Here's how the part is built. I have some questions about the finished solid (model axes, mm). Round coordinates to 2 decimals unless told otherwise and drop trailing zeros. Write each loop counter-clockwise with the first axis right and the second up, starting at its lowest first coordinate (ties: lowest second). Pieces come first, ordered by that corner, then holes. Notation, with made-up numbers: (51.5, 28.5) - (91.5, 28.5) arc R19 ccw to (91.5, 40.5) - close; hole circle Ø6 at (87, 88). An arc over 180 degrees is marked (long way). One line per item, written item: value. Start each with the question number.
Item 1: Imagine slicing it at A-A, the plane x = 0. Please give me the cut outline in (y, z), then the cut area to 3 significant figures.
Item 2: For P1, Ø4, axis at x = -10, z = 3, coming from the -Y side; P2, Ø3, axis at y = -8.5, z = 0, coming from the +X side; P3, Ø2, axis at x = 1, y = -11, coming from the +Z side, each with a flat end and sliding along its axis, tell me the tip position at first contact or that it passes through.
Item 3: Imagine slicing it at C-C, the plane z = -7. Please give me the cut outline in (x, y), then the cut area to 3 significant figures.
Item 4: Thinking about a two-plate mould opening in Y: for faces 1 (the face through (-7.78, 4.05, -10.34)), 2 (the face through (-10.144, -2.253, -11.037)), 3 (the face through (-6, -6, -1.149)), which applies, released by +Y, released by -Y, zero draft, split by the parting line, or undercut?
Item 5: If I drill on line 1 (Z direction, x = 18, y = 13.5); line 2 (X direction, y = 1, z = -15.5); line 3 (Y direction, x = -7, z = -20.5), over which ranges is the centre line in solid material (lowest first)?
Item 6: Imagine slicing it at D-D, the plane z = 9.5. Please give me the cut outline in (x, y).
Autodesk Inventor part; units mm, degrees
ref_plane "YZ Plane" through (0, 0, 0) normal (1, 0, 0) x (0, 1, 0)
ref_plane "XZ Plane" through (0, 0, 0) normal (0, 1, 0) x (-1, 0, 0)
ref_plane "XY Plane" through (0, 0, 0) normal (0, 0, 1) x (1, 0, 0)
sketch "Sketch1" plane through (0, 0, 0) normal (1, 0, 0) x (0, 1, 0)
  line L0 (22, 22.8504) -> (6, 0)
  line L1 (6, 0) -> (13, -26.1244)
  line L2 (13, -26.1244) -> (14.4343, -26.1244)
  line L3 (14.4343, -26.1244) -> (7.7423, -1.1493)
  line L4 (7.7423, -1.1493) -> (24, -1.1493)
  line L5 (22, 22.8504) -> (24, 22.8504)
  line L6 (24, 22.8504) -> (24, -1.1493)
  line L7 (0, 0) -> (6, 0) construction
  line L8 (0, 0) -> (0, 52.5591) construction
  dimension "d1" = 105
  dimension "d2" = 105
  dimension "d3" = 24
  dimension "d4" = 22
  dimension "d5" = 13
  dimension "d6" = 35
  dimension "d8" = 6
  dimension "d9" = 23.9997
  dimension "d10" = 7.181
  dimension "d11" = 29.7087
revolve "Revolution1" add sketch "Sketch1" angle 360 about axis through (0, 0, 0) along (0, 0, 1)
properties part number "nozzle"
Values follow:
1. outline: (-24, -1.15) - (-7.74, -1.15) - (-14.43, -26.12) - (-13, -26.12) - (-6, 0) - (-22, 22.85) - (-24, 22.85) - close; (6, 0) - (13, -26.12) - (14.43, -26.12) - (7.74, -1.15) - (24, -1.15) - (24, 22.85) - (22, 22.85) - close
1. area: 570 mm^2
2. P1: stops at y = -22.63
2. P2: stops at x = 22.96
2. P3: stops at z = 8.63
3. outline: circle Ø18.62 at (0, 0); hole circle Ø15.75 at (0, 0)
3. area: 77.4 mm^2
4. face 1: undercut
4. face 2: split by the parting line
4. face 3: zero draft
5. line 1: z = -1.15 to 22.85
5. line 2: x = -11.54 to -10.1, 10.1 to 11.54
5. line 3: y = -10.87 to -9.12, 9.12 to 10.87
6. outline: circle Ø48 at (0, 0); hole circle Ø25.3 at (0, 0)
